```python
from build123d import *
from build123d import SkipClean  # not in build123d's __all__

# Parameters (mm, degrees)
F1_DEPTH = 30
F3_START = -5
F2_R     = 2.5
F3_DEPTH = 20


with BuildPart() as f1:
    # F0 (on Front) → F1 (new body)
    with BuildSketch(Plane.XZ):
        with BuildLine():
            ThreePointArc((-2, 1.5), (-0.790569415, -2.3717082451), (2.5, 0))
            ThreePointArc((2.5, 0), (2.3717082451, 0.790569415), (2, 1.5))
            Line((2, 1.5), (-2, 1.5))
        make_face()
    extrude(amount=F1_DEPTH)

    # F2 (on face) → F3 (join)
    with BuildSketch(Plane.XZ.offset(30).offset(F3_START)):
        Circle(F2_R)
    with SkipClean():  # cleaning this boolean's faces spoils the solid; the shape is the same uncleaned
        extrude(amount=-F3_DEPTH)


solid = f1.part
```
Verification items for the finished model (mm, model axes). A direction names the side the tool comes from. Give positions to 0.01 mm unless a question says otherwise; leave off trailing zeros. Loops run counter-clockwise (first coordinate to the right, second up) from the corner with the lowest first, then second, coordinate; pieces in that order, holes last. Notation, with made-up numbers: M -33,4.25 L 6,4.25 A25 cw 6,37.25 Z; hole C 61,39 d9. An arc over 180 degrees is marked long. One line per question, with ' | ' between items.
Item 1: Depth check by flat-ended pin: P1, Ø2, axis at x = 1, y = -3.5, coming from the +Z side; P2, Ø1.5, axis at x = -1.5, y = -15, coming from the +Z side; P3, Ø2, axis at y = -12.5, z = 1.5, coming from the -X side. Enter the tip coordinate at first touch or a pass-through.
Completed:
P1: stops at z = 1.5 | P2: stops at z = 2.38 | P3: stops at x = -2.45
Item 2: Section check B-B, the plane y = -25.5. Record the cut outline in (x, z).
Completed:
outline: M -2,1.5 A2.5 ccw long 2,1.5 Z
Item 3: Tool access check on faces 1 (the face through (0, -30, 0)), 2 (the face through (0, -5, 2)), 3 (the face through (0, -25, 2)). Record the directions out of +Z, -Z, +X, -X, +Y, -Y that give a thin tool (end or side, any length) a straight path to the whole face; none if there is none.
Completed:
face 1: +Z, -Z, +X, -X, -Y | face 2: +Z, +X, -X, +Y | face 3: +Z, +X, -X, -Y
Item 4: Section check A-A, the plane x = 0. Record the cut outline in (y, z), plus the area to 3 significant figures.
Completed:
outline: M -30,-2.5 L 0,-2.5 L 0,1.5 L -5,1.5 L -5,2.5 L -25,2.5 L -25,1.5 L -30,1.5 Z | area: 140 mm^2
Item 5: Section check D-D, the plane z = 0.75. Record the cut outline in (x, y), plus the area to 3 significant figures.
Completed:
outline: M -2.38,-30 L 2.38,-30 L 2.38,0 L -2.38,0 Z | area: 143 mm^2
Item 6: Section check C-C, the plane x = -1.3. Record the cut outline in (y, z).
Completed:
outline: M -30,-2.14 L 0,-2.14 L 0,1.5 L -5,1.5 L -5,2.14 L -25,2.14 L -25,1.5 L -30,1.5 Z
Item 7: Thickness scan on line 1 (X direction, y = -3, z = 1.15); line 2 (X direction, y = -4.5, z = 1.35). Record the ranges inside material, lowest first. Write a range as [from, to].
Completed:
line 1: x = [-2.22, 2.22] | line 2: x = [-2.1, 2.1]
